Read the model definition and answer for the solid it produces. Units are mm, in the model's axes. A direction names the side the tool comes from. Round coordinates to 2 decimals unless told otherwise and drop trailing zeros. Order: outer loops, then holes, each group sorted by start corner. A loop starts at its lowest first (then second) coordinate and runs counter-clockwise, first axis right, second up.
from build123d import *

# Parameters (mm, degrees)
F0_W     = 191.1350041628
F0_H     = 103.0816659331
F0_W_2   = 170.391663909
F0_H_2   = 81.4916715026
F1_DEPTH = 101.6
F2_W     = 84.5615752041
F2_H     = 10.7949972153
F3_DEPTH = 44.45
F4_W     = 84.5615752041
F4_H     = 10.7949972153
F5_DEPTH = 44.45
F6_R     = 12.9453213724
F7_DEPTH = 25.4
F8_R     = 12.9608479871
F9_DEPTH = 25.4


with BuildPart() as f1:
    # F0 (on Top) → F1 (new body)
    with BuildSketch(Plane.XY):
        Rectangle(F0_W, F0_H)
        Rectangle(F0_W_2, F0_H_2, mode=Mode.SUBTRACT)
    extrude(amount=F1_DEPTH)

    # F2 (on face) → F3 (cut)
    with BuildSketch(Plane.XY.offset(101.6)):
        with Locations((-1.3613607734, -46.1433343589)):
            Rectangle(F2_W, F2_H)
    extrude(amount=-F3_DEPTH, mode=Mode.SUBTRACT)

    # F4 (on face) → F5 (cut)
    with BuildSketch(Plane.XY.offset(101.6)):
        with Locations((-1.3613607734, 46.1433343589)):
            Rectangle(F4_W, F4_H)
    extrude(amount=-F5_DEPTH, mode=Mode.SUBTRACT)

    # F6 (on face) → F7 (cut)
    with BuildSketch(Plane(origin=(-95.5675020814, 0, 0), x_dir=(0, -1, 0), z_dir=(-1, 0, 0))):
        with Locations((0, 57.6301626861)):
            Circle(F6_R)
    extrude(amount=-F7_DEPTH, mode=Mode.SUBTRACT)

    # F8 (on face) → F9 (cut)
    with BuildSketch(Plane.YZ.offset(95.5675020814)):
        with Locations((0, 50.8931577206)):
            Circle(F8_R)
    extrude(amount=-F9_DEPTH, mode=Mode.SUBTRACT)


solid = f1.part
Q1. A cutting plane is placed at D-D, the plane y = 44. Give the vertices of the cut face in (x, z).
Outcome:
outline: (-95.57, 0) - (95.57, 0) - (95.57, 101.6) - (40.92, 101.6) - (40.92, 57.15) - (-43.64, 57.15) - (-43.64, 101.6) - (-95.57, 101.6) - close
Q2. A cutting plane is placed at B-B, the plane x = -14. Give the vertices of the cut face in (y, z), plus the area to 3 significant figures.
Outcome:
outline: (-51.54, 0) - (-40.75, 0) - (-40.75, 57.15) - (-51.54, 57.15) - close; (40.75, 0) - (51.54, 0) - (51.54, 57.15) - (40.75, 57.15) - close
area: 1,230 mm2
Q3. Flat-ended cylindrical pins translate along their axes: pin 1 (3 mm diameter, centred on x = 17.5, y = -47.5, fed in from +Z); pin 2 (12 mm diameter, centred on x = 57, y = 31.5, fed in from +Z). Find the tip coordinate at first contact, or state that the pin passes through.
Outcome:
pin 1: stops at z = 57.15
pin 2: passes through
Q4. A cutting plane is placed at C-C, the plane z = 68.5. Give the vertices of the cut face in (x, y), plus the area to 3 significant figures.
Outcome:
outline: (-95.57, -51.54) - (-43.64, -51.54) - (-43.64, -40.75) - (-85.2, -40.75) - (-85.2, -7.03) - (-95.57, -7.03) - close; (-95.57, 7.03) - (-85.2, 7.03) - (-85.2, 40.75) - (-43.64, 40.75) - (-43.64, 51.54) - (-95.57, 51.54) - close; (40.92, -51.54) - (95.57, -51.54) - (95.57, 51.54) - (40.92, 51.54) - (40.92, 40.75) - (85.2, 40.75) - (85.2, -40.75) - (40.92, -40.75) - close
area: 3,850 mm2
Q5. For a pull along Z with two mould halves and no side action, classify faces 1 (the face through (90.454, 5.981, 39.395)), 2 (the face through (-87, 1, 101.6)), 3 (the face through (-1, -51.541, 50)) as released by +Z, released by -Z, zero draft, split by the parting line, or undercut.
Outcome:
face 1: undercut
face 2: released by +Z
face 3: zero draft
Q6. For faces 4 (the face through (-1, 40.746, 39)), 5 (the face through (-90.454, 2.806, 44.993)), 6 (the face through (-43.642, 46, 80)), determine the directions among +Z, -Z, +X, -X, +Y, -Y from which every point of the face is accessible in a straight line to the end or side of a thin tool.
Outcome:
face 4: +Z, -Z
face 5: -X
face 6: +Z, +Y, -Y
Q7. A cutting plane is placed at A-A, the plane y = 0. Give the vertices of the cut face in (x, z).
Outcome:
outline: (-95.57, 0) - (-85.2, 0) - (-85.2, 44.68) - (-95.57, 44.68) - close; (-95.57, 70.58) - (-85.2, 70.58) - (-85.2, 101.6) - (-95.57, 101.6) - close; (85.2, 0) - (95.57, 0) - (95.57, 37.93) - (85.2, 37.93) - close; (85.2, 63.85) - (95.57, 63.85) - (95.57, 101.6) - (85.2, 101.6) - close
Q8. Straight lines are drawn through the part: probe 1 along X at (y, z) = (-43, 86); probe 2 along X at (y, z) = (-17, 40.5); probe 3 along Y at (x, z) = (68.5, 13). For each, find the intervals that lie inside material, in ascending order.
Outcome:
probe 1: x = -95.57 to -43.64, 40.92 to 95.57
probe 2: x = -95.57 to -85.2, 85.2 to 95.57
probe 3: y = -51.54 to -40.75, 40.75 to 51.54
